```python
from build123d import *

# Parameters (mm, degrees)
SKETCH1_W            = 175
SKETCH1_H            = 60
BOSS_EXTRUDE1_DEPTH  = 25
SKETCH2_W            = 172.037419054
SKETCH2_H            = 56.878309912
CUT_EXTRUDE2_DEPTH   = 23
CUT_EXTRUDE4_DEPTH   = 180.30421077
SKETCH5_W            = 56.619672169
SKETCH5_H            = 2.543260903
BOSS_EXTRUDE2_DEPTH  = 140
BOSS_EXTRUDE3_DEPTH  = 2
SKETCH7_R            = 4.069899946
SKETCH7_R_2          = 3.573578561
BOSS_EXTRUDE4_DEPTH  = 5
BOSS_EXTRUDE6_DEPTH  = 2
SKETCH9_R            = 3.803746222
BOSS_EXTRUDE7_DEPTH  = 2
SKETCH10_R           = 2.430826278
BOSS_EXTRUDE8_DEPTH  = 5
SKETCH11_R           = 1.370011297
SKETCH11_R_2         = 1.313817757
SKETCH11_R_3         = 1.331167219
BOSS_EXTRUDE9_DEPTH  = 2
SKETCH12_R           = 0.613636394
SKETCH12_R_2         = 0.736542168
SKETCH12_R_3         = 0.775004172
BOSS_EXTRUDE10_DEPTH = 2


with BuildPart() as part:
    # Sketch1 → Boss-Extrude1 (new body)
    with BuildSketch(Plane(origin=(0, 0, 0), x_dir=(1, 0, 0), z_dir=(0, 1, 0))):
        Rectangle(SKETCH1_W, SKETCH1_H)
    extrude(amount=BOSS_EXTRUDE1_DEPTH)

    # Sketch2 → Cut-Extrude2 (cut)
    with BuildSketch(Plane(origin=(0, 25, 0), x_dir=(1, 0, 0), z_dir=(0, 1, 0))):
        Rectangle(SKETCH2_W, SKETCH2_H)
    extrude(amount=-CUT_EXTRUDE2_DEPTH, mode=Mode.SUBTRACT)

    # Sketch3 → Cut-Extrude4 (cut, through all)
    with BuildSketch(Plane(origin=(87.5, 0, 0), x_dir=(0, 0, -1), z_dir=(1, 0, 0))):
        with BuildLine():
            ThreePointArc((-22.681609782, 25), (-20.139304377, 21.416181436), (-19.241971202, 17.114801954))
            Line((-19.241971202, 17.114801954), (19.672994279, 17.951296347))
            ThreePointArc((19.672994279, 17.951296347), (20.393002527, 21.739785058), (22.452628009, 25))
            Line((22.452628009, 25), (-22.681609782, 25))
        make_face()
    extrude(amount=-CUT_EXTRUDE4_DEPTH, mode=Mode.SUBTRACT)

    # Sketch5 → Boss-Extrude2 (add)
    with BuildSketch(Plane(origin=(-86.018709527, 0, 0), x_dir=(0, 0, -1), z_dir=(1, 0, 0))):
        with Locations((0.129318872, 13.450991009)):
            Rectangle(SKETCH5_W, SKETCH5_H)
    extrude(amount=BOSS_EXTRUDE2_DEPTH)

    # Sketch6 → Boss-Extrude3 (add)
    with BuildSketch(Plane(origin=(87.5, 0, 0), x_dir=(0, 0, -1), z_dir=(1, 0, 0))):
        with BuildLine():
            Line((-23.739887735, 12.934037749), (-14.749940356, 12.934037749))
            ThreePointArc((-14.749940356, 12.934037749), (-14.474436425, 12.796150035), (-14.296501276, 12.544645521))
            Line((-14.296501276, 12.544645521), (-14.296501276, 2.814596709))
            ThreePointArc((-14.296501276, 2.814596709), (-14.348088202, 2.742066754), (-14.427356599, 2.701590504))
            Line((-14.427356599, 2.701590504), (-23.96895697, 2.701590504))
            ThreePointArc((-23.96895697, 2.701590504), (-24.058326953, 2.766456684), (-24.077974584, 2.875124001))
            Line((-24.077974584, 2.875124001), (-24.077974584, 12.450209245))
            ThreePointArc((-24.077974584, 12.450209245), (-24.000062189, 12.755803504), (-23.739887735, 12.934037749))
        make_face()
    extrude(amount=BOSS_EXTRUDE3_DEPTH)

    # Sketch7 → Boss-Extrude4 (add)
    with BuildSketch(Plane(origin=(89.5, 0, 0), x_dir=(0, 0, -1), z_dir=(1, 0, 0))):
        with Locations((-18.991835841, 7.548541402)):
            Circle(SKETCH7_R)
        with Locations((-18.991835841, 7.548541402)):
            Circle(SKETCH7_R_2, mode=Mode.SUBTRACT)
    extrude(amount=BOSS_EXTRUDE4_DEPTH)

    # Sketch8 → Boss-Extrude6 (add)
    with BuildSketch(Plane(origin=(89.5, 0, 0), x_dir=(0, 0, -1), z_dir=(1, 0, 0))):
        Polygon((-22.791586736, 11.211896935), (-22.48659006, 11.74204685), (-22.793215015, 12.271256677), (-23.404836647, 12.27031659), (-23.709833324, 11.740166675), (-23.403208368, 11.210956848), align=None)
        Polygon((-15.214334729, 11.35367817), (-14.921128157, 11.882675416), (-15.232649924, 12.40109838), (-15.837378264, 12.390524097), (-16.130584836, 11.861526851), (-15.819063069, 11.343103888), align=None)
        Polygon((-22.614375311, 3.648960977), (-22.903289414, 4.149374881), (-23.481117618, 4.149374881), (-23.770031721, 3.648960977), (-23.481117618, 3.148547073), (-22.903289414, 3.148547073), align=None)
        Polygon((-14.98393783, 3.084271685), (-14.687192917, 3.521636864), (-14.917589816, 3.997308087), (-15.444731629, 4.035614131), (-15.741476542, 3.598248952), (-15.511079643, 3.122577729), align=None)
    extrude(amount=BOSS_EXTRUDE6_DEPTH)

    # Sketch9 → Boss-Extrude7 (add)
    with BuildSketch(Plane(origin=(87.5, 0, 0), x_dir=(0, 0, -1), z_dir=(1, 0, 0))):
        with Locations(Location((4.287117765, 9.151764618, 0), (0, 0, 180))):
            Circle(SKETCH9_R)
    extrude(amount=BOSS_EXTRUDE7_DEPTH)

    # Sketch10 → Boss-Extrude8 (add)
    with BuildSketch(Plane(origin=(89.5, 0, 0), x_dir=(0, 0, -1), z_dir=(1, 0, 0))):
        with Locations((4.363010591, 8.979818711)):
            Circle(SKETCH10_R)
    extrude(amount=BOSS_EXTRUDE8_DEPTH)

    # Sketch11 → Boss-Extrude9 (add)
    with BuildSketch(Plane(origin=(87.5, 0, 0), x_dir=(0, 0, -1), z_dir=(1, 0, 0))):
        with Locations(Location((24.040397356, 12.193405529, 0), (0, 0, 180))):
            Circle(SKETCH11_R)
        with Locations(Location((24.040397356, 8.016708701, 0), (0, 0, 180))):
            Circle(SKETCH11_R_2)
        with Locations(Location((24.040397356, 4.159285121, 0), (0, 0, 180))):
            Circle(SKETCH11_R_3)
    extrude(amount=BOSS_EXTRUDE9_DEPTH)

    # Sketch12 → Boss-Extrude10 (add)
    with BuildSketch(Plane(origin=(89.5, 0, 0), x_dir=(0, 0, -1), z_dir=(1, 0, 0))):
        with Locations((24.040397356, 12.144680604)):
            Circle(SKETCH12_R)
        with Locations((24.040397356, 8.016708701)):
            Circle(SKETCH12_R_2)
        with Locations((23.993599031, 4.133922204)):
            Circle(SKETCH12_R_3)
    extrude(amount=BOSS_EXTRUDE10_DEPTH)


solid = part.part
```
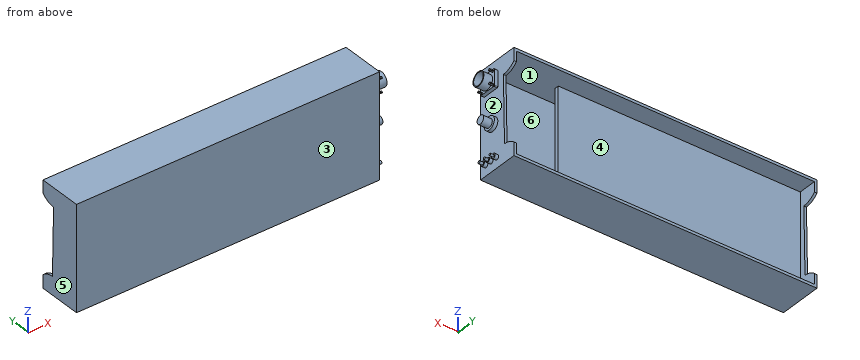
Geometry check sheet. Reference: the model listing, model coordinates, mm. Face numbers are marked on the shaded views. A direction names the side the tool comes from. Round coordinates to 2 decimals unless told otherwise and drop trailing zeros. Loops run counter-clockwise (first coordinate to the right, second up) from the corner with the lowest first, then second, coordinate; pieces in that order, holes last. Notation, with made-up numbers: (70.25, 42) - (99.25, 42) arc R18 cw to (99.25, 69) - close; hole circle Ø2 at (64, 65). An arc over 180 degrees is marked (long way). Write item = value, one per line. Start each with the question number.
1. Mould release check, pull along X, two halves, no side actions. Record for the marked faces 1, 2 and 3: released by +X, released by -X, zero draft, split by the parting line, or undercut.
2. Section check C-C on z = 4. Enter the section's corners in (x, y), then the cut area to 3 significant figures.
3. Set-up check for the marked faces 4, 5 and 6: record each of +Z, -Z, +X, -X, +Y, -Y from which the full face is reachable in a straight line by a thin tool's end or side.
4. Section check D-D on x = 56.5. Enter the section's corners in (y, z).
5. Thickness scan on line 1 (Y direction, x = -78.5, z = -13.5); line 2 (X direction, y = 14, z = -17); line 3 (Z direction, x = -9.5, y = 15). Record the ranges inside material, lowest first.
6. Section check A-A on y = 20.75. Enter the section's corners in (x, z).
7. Section check B-B on x = -10.5. Enter the section's corners in (y, z), then the cut area to 3 significant figures.
8. Depth check by flat-ended pin: pin 1 (0.6 mm diameter, centred on x = 88, z = 21.5, fed in from -Y); pin 2 (1 mm diameter, centred on x = 89, y = 7.5, fed in from -Z); pin 3 (1.3 mm diameter, centred on y = 8, z = -24, fed in from +X); pin 4 (6 mm diameter, centred on x = 14, z = 14, fed in from -Y). Enter the tip coordinate at first touch or a pass-through.
Working result:
q1.face_1 = undercut
q1.face_2 = released by +X
q1.face_3 = zero draft
q2.outline = (-87.5, 0) - (87.5, 0) - (87.5, 17.44) - (86.02, 17.44) - (86.02, 2) - (-86.02, 2) - (-86.02, 12.18) - (53.98, 12.18) - (53.98, 14.72) - (-86.02, 14.72) - (-86.02, 17.44) - (-87.5, 17.44) - close
q2.area = 752 mm^2
q3.face_4 = +Y
q3.face_5 = +Z, -Z, -X, +Y, -Y
q3.face_6 = none
q4.outline = (0, -30) - (25, -30) - (25, -28.44) - (2, -28.44) - (2, 28.44) - (25, 28.44) - (25, 30) - (0, 30) - close
q5.line_1 = 0 to 2, 12.18 to 14.72
q5.line_2 = -87.5 to 53.98, 86.02 to 87.5
q5.line_3 = -30 to -28.44, 28.44 to 30
q6.outline = (-87.5, -30) - (87.5, -30) - (87.5, -20.06) - (86.02, -20.06) - (86.02, -28.44) - (-86.02, -28.44) - (-86.02, -20.06) - (-87.5, -20.06) - close; (-87.5, 19.87) - (-86.02, 19.87) - (-86.02, 28.44) - (86.02, 28.44) - (86.02, 19.87) - (87.5, 19.87) - (87.5, 30) - (-87.5, 30) - close
q7.outline = (0, -30) - (25, -30) - (25, -28.44) - (14.72, -28.44) - (14.72, 28.18) - (12.18, 28.18) - (12.18, -28.44) - (2, -28.44) - (2, 28.44) - (25, 28.44) - (25, 30) - (0, 30) - close
q7.area = 336 mm^2
q8.pin_1 = 2.7
q8.pin_2 = -25.35
q8.pin_3 = 91.5
q8.pin_4 = 0
